The listing builds one solid part. Answer for the finished solid, in the listing's coordinates (mm). A direction names the side the tool comes from. Round coordinates to 2 decimals unless told otherwise and drop trailing zeros. Loops run counter-clockwise (first coordinate to the right, second up) from the corner with the lowest first, then second, coordinate; pieces in that order, holes last. Notation, with made-up numbers: (26, 40.5) -> (82, 40.5) arc R24 ccw to (82, 58.5) -> close; hole circle Ø5 at (19, -33.75). An arc over 180 degrees is marked (long way). Use a Markdown table: item, result. Add a question column.
Q1. Section B-B on x = 14 is taken. Give the vertices of the cut face in (y, z), then the cut area to 3 significant figures.
Q2. For a pull along X with two mould halves and no side action, classify faces 4 (the flat face through (-5, 8, 9.435)), 5 (the cylindrical face through (44.51, 6.83, 8.94)), 6 (the cylindrical face through (43.1, 79.35, 8.42)) as released by +X, released by -X, zero draft, split by the parting line, or undercut.
Q3. Which of the six approach directions +Z, -Z, +X, -X, +Y, -Y give full straight-line access (tool end or side, diameter ignored) to faces 1 (the flat face through (-5, 8, 7.435)), 2 (the cylindrical face through (-48.592, 35.557, 8.449)), 3 (the flat face through (49, 81, 8.435))?
Q4. Given pin 1 Ø2.5 at (x, y) = (-25.49, 6.2) entering from +Z; pin 2 Ø3 at (x, y) = (47, 5.5) entering from +Z, each flat-ended and moving along its own axis, determine where each tip first touches the part or whether it passes through.
Q5. Section C-C on z = 8.1 is taken. Give the number of separate pieces and of enclosed holes in the cut face, then the cut area to 3 significant figures.
Q6. Section A-A on y = 75 is taken. Give the vertices of the cut face in (x, z), then the cut area to 3 significant figures.
Q7. Consider line 1 (X direction, y = 64.5, z = 8.05); line 2 (Y direction, x = 9.5, z = 9.2); line 3 (Y direction, x = 47.5, z = 8.6). Determine where each line is inside the solid, lowest interval first.
from build123d import *

# Parameters (mm, degrees)
SKETCH1_W                  = 109.5
SKETCH1_H                  = 82.5
BOSS_EXTRUDE1_DEPTH        = 2
F_3_5_3_5_DIAMETER_HOLE1_D = 3.5
F_2_2_2_2_DIAMETER_HOLE1_D = 2.2
SKETCH12_R                 = 3
CUT_EXTRUDE1_DEPTH         = 1
FILLET1_R                  = 3
FILLET2_R                  = 1


with BuildPart() as part:
    # Sketch1 → Boss-Extrude1 (new body)
    with BuildSketch(Plane.XY.offset(7.43465612)):
        with Locations((-0.743641502, 44.70185693)):
            Rectangle(SKETCH1_W, SKETCH1_H)
        with BuildLine():
            Line((-45.493641502, 34.70185693), (-49.493641502, 34.70185693))
            Line((-49.493641502, 34.70185693), (-49.493641502, 54.70185693))
            Line((-49.493641502, 54.70185693), (-45.493641502, 54.70185693))
            Line((-45.493641502, 54.70185693), (-45.493641502, 77.20185693))
            ThreePointArc((-45.493641502, 77.20185693), (-44.614961845, 79.323177274), (-42.493641502, 80.20185693))
            Line((-42.493641502, 80.20185693), (41.006358498, 80.20185693))
            ThreePointArc((41.006358498, 80.20185693), (43.127678842, 79.323177274), (44.006358498, 77.20185693))
            Line((44.006358498, 77.20185693), (44.006358498, 54.70185693))
            Line((44.006358498, 54.70185693), (48.006358498, 54.70185693))
            Line((48.006358498, 54.70185693), (48.006358498, 44.70185693))
            Line((48.006358498, 44.70185693), (48.006358498, 34.70185693))
            Line((48.006358498, 34.70185693), (44.006358498, 34.70185693))
            Line((44.006358498, 34.70185693), (44.006358498, 12.20185693))
            ThreePointArc((44.006358498, 12.20185693), (43.127678842, 10.080536587), (41.006358498, 9.20185693))
            Line((41.006358498, 9.20185693), (-42.493641502, 9.20185693))
            ThreePointArc((-42.493641502, 9.20185693), (-44.614961845, 10.080536587), (-45.493641502, 12.20185693))
            Line((-45.493641502, 12.20185693), (-45.493641502, 34.70185693))
        make_face(mode=Mode.SUBTRACT)
    extrude(amount=BOSS_EXTRUDE1_DEPTH)

    # Ø3.5 (3.5) Diameter Hole1 (through all)
    with Locations(Plane.XY.offset(9.43465612)):
        with Locations((-48.993641502, 6.70185693), (-48.993641502, 82.70185693), (47.506358498, 82.70185693), (47.506358498, 6.70185693)):
            Hole(F_3_5_3_5_DIAMETER_HOLE1_D / 2)

    # Ø2.2 (2.2) Diameter Hole1 (through all)
    with Locations(Plane(origin=(-25.493641502, 83.20185693, 9.43465612), x_dir=(1, 0, 0), z_dir=(0, 0, 1))):
        with Locations((0, 0), (49.5, 0), (49.5, -77), (0, -77)):
            Hole(F_2_2_2_2_DIAMETER_HOLE1_D / 2)

    # Sketch12 → Cut-Extrude1 (cut)
    with BuildSketch(Plane.XY.offset(9.43465612)):
        with Locations((-48.993641502, 82.70185693)):
            Circle(SKETCH12_R)
        with Locations((47.506358498, 82.70185693)):
            Circle(SKETCH12_R)
        with Locations((47.506358498, 6.70185693)):
            Circle(SKETCH12_R)
        with Locations((-48.993641502, 6.70185693)):
            Circle(SKETCH12_R)
    extrude(amount=-CUT_EXTRUDE1_DEPTH, mode=Mode.SUBTRACT)

    # Fillet1
    fillet1_edges = [part.edges().sort_by_distance(p)[0] for p in [
        (48.006358498, 34.70185693, 8.43465612),
        (48.006358498, 54.70185693, 8.43465612),
        (-49.493641502, 54.70185693, 8.43465612),
        (-49.493641502, 34.70185693, 8.43465612),
    ]]
    fillet(fillet1_edges, radius=FILLET1_R)

    # Fillet2
    fillet2_edges = [part.edges().sort_by_distance(p)[0] for p in [
        (44.006358498, 34.70185693, 8.43465612),
        (44.006358498, 54.70185693, 8.43465612),
        (-45.493641502, 34.70185693, 8.43465612),
        (-45.493641502, 54.70185693, 8.43465612),
    ]]
    fillet(fillet2_edges, radius=FILLET2_R - 0.0001)  # a hair under: the kernel refuses the full size


solid = part.part
Checked values:
| question | item | result |
|---|---|---|
| 1 | outline | (3.45, 7.43) -> (9.2, 7.43) -> (9.2, 9.43) -> (3.45, 9.43) -> close; (80.2, 7.43) -> (85.95, 7.43) -> (85.95, 9.43) -> (80.2, 9.43) -> close |
| 1 | area | 23.0 mm2 |
| 2 | face 4 | zero draft |
| 2 | face 5 | undercut |
| 2 | face 6 | undercut |
| 3 | face 1 | -Z, +X, -X, +Y, -Y |
| 3 | face 2 | +Z, -Z |
| 3 | face 3 | +Z |
| 4 | pin 1 | stops at z = 9.43 |
| 4 | pin 2 | stops at z = 8.43 |
| 5 | separate pieces | 1 |
| 5 | enclosed holes | 9 |
| 5 | area | 2,480 mm2 |
| 6 | outline | (-55.49, 7.43) -> (-45.49, 7.43) -> (-45.49, 9.43) -> (-55.49, 9.43) -> close; (44.01, 7.43) -> (54.01, 7.43) -> (54.01, 9.43) -> (44.01, 9.43) -> close |
| 6 | area | 40.0 mm2 |
| 7 | line 1 | x = -55.49 to -45.49, 44.01 to 54.01 |
| 7 | line 2 | y = 3.45 to 9.2, 80.2 to 85.95 |
| 7 | line 3 | y = 3.45 to 3.7, 9.7 to 36.03, 53.37 to 79.7, 85.7 to 85.95 |
